Geometry: final body of the model. Coordinates: model frame, mm. A direction names the side the tool comes from. Round coordinates to 2 decimals unless told otherwise and drop trailing zeros. Loops run counter-clockwise (first coordinate to the right, second up) from the corner with the lowest first, then second, coordinate; pieces in that order, holes last. Notation, with made-up numbers: (-37.5, -6.75) - (13.5, -6.75) arc R18 ccw to (13.5, 15.25) - close; hole circle Ø11 at (77.25, -33.75). An arc over 180 degrees is marked (long way). Answer as CSV lines item,"result".
from build123d import *

# Parameters (mm, degrees)
SKETCH_1_R      = 2.1
EXTRUDE_1_DEPTH = 3
SKETCH_2_R      = 14
EXTRUDE_2_DEPTH = 8
SKETCH_3_R      = 11
EXTRUDE_3_DEPTH = 3
FILLET_1_R      = 2
FILLET_2_R      = 1


with BuildPart() as part:
    # 草图1 → 凸台-拉伸1 (new body)
    with BuildSketch(Plane.XY):
        with BuildLine():
            Line((-22.192307692, 4.213250442), (-8.346153846, 13.061076371))
            ThreePointArc((-8.346153846, 13.061076371), (0, 15.5), (8.346153846, 13.061076371))
            Line((8.346153846, 13.061076371), (22.192307692, 4.213250442))
            ThreePointArc((22.192307692, 4.213250442), (24.5, 0), (22.192307692, -4.213250442))
            Line((22.192307692, -4.213250442), (8.346153846, -13.061076371))
            ThreePointArc((8.346153846, -13.061076371), (0, -15.5), (-8.346153846, -13.061076371))
            Line((-8.346153846, -13.061076371), (-22.192307692, -4.213250442))
            ThreePointArc((-22.192307692, -4.213250442), (-24.5, 0), (-22.192307692, 4.213250442))
        make_face()
        with Locations((-19.5, 0)):
            Circle(SKETCH_1_R, mode=Mode.SUBTRACT)
        with Locations((19.5, 0)):
            Circle(SKETCH_1_R, mode=Mode.SUBTRACT)
    extrude(amount=EXTRUDE_1_DEPTH)

    # 草图2 → 凸台-拉伸2 (add)
    with BuildSketch(Plane.XY.offset(3)):
        Circle(SKETCH_2_R)
    extrude(amount=EXTRUDE_2_DEPTH)

    # 草图3 → 凸台-拉伸3 (add)
    with BuildSketch(Plane.XY.offset(11)):
        Circle(SKETCH_3_R)
    extrude(amount=EXTRUDE_3_DEPTH)

    # 草图4 → 切除-旋转1 (revolve, cut)
    with BuildSketch(Plane(origin=(0, 0, 0), x_dir=(0, 0, -1), z_dir=(1, 0, 0))):
        with BuildLine():
            Line((-18, 0), (-4, 0))
            ThreePointArc((-4, 0), (-11, 7), (-18, 0))
        make_face()
    revolve(axis=Axis((0, 0, 18), (0, 0, -1)), mode=Mode.SUBTRACT)

    # 圆角1
    fillet_1_edges = [part.edges().sort_by_distance(p)[0] for p in [
        (-14, 0, 11),
    ]]
    fillet(fillet_1_edges, radius=FILLET_1_R)

    # 圆角2
    fillet_2_edges = [part.edges().sort_by_distance(p)[0] for p in [
        (-11, 0, 14),
    ]]
    fillet(fillet_2_edges, radius=FILLET_2_R)


solid = part.part
(1) Access query for faces 1 (the face through (12.932, -5.362, 5.958)), 2 (the face through (0, 0, 0)). Directions: +Z, -Z, +X, -X, +Y, -Y. A direction counts if a zero-diameter tool reaches every point of the face in a straight line with its end or side. Return the directions, or none.
Findings below:
face 1,"+Z"
face 2,"-Z, +X, -X, +Y, -Y"
(2) Section A-A (z = 2.5). Output: boundary loops of the cut face in (x, y), and give its area (3 significant figures).
Findings below:
outline,"(-22.19, -4.21) - (-8.35, -13.06) arc R15.5 ccw to (8.35, -13.06) - (22.19, -4.21) arc R5 ccw to (22.19, 4.21) - (8.35, 13.06) arc R15.5 ccw to (-8.35, 13.06) - (-22.19, 4.21) arc R5 ccw to start; hole circle Ø4.2 at (-19.5, 0); hole circle Ø4.2 at (19.5, 0)"
area,"969 mm2"
(3) Section B-B (x = -19.5). Output: boundary loops of the cut face in (y, z).
Findings below:
outline,"(-5.93, 0) - (-2.1, 0) - (-2.1, 3) - (-5.93, 3) - close; (2.1, 0) - (5.93, 0) - (5.93, 3) - (2.1, 3) - close"
(4) Pin query (flat end, axial travel): P1, Ø1, axis at x = -11, z = 6.5, coming from the -Y side; P2, Ø5.5, axis at x = 19.5, y = 0, coming from the +Z side; P3, Ø3, axis at y = -10, z = 10, coming from the -X side; P4, Ø4, axis at x = -19.5, y = 0, coming from the -Z side. Return the tip coordinate at first contact, or that it passes through.
Findings below:
P1,"y = -9.26"
P2,"z = 3"
P3,"x = -10.98"
P4,"through"
(5) Material intervals for line 1 along Y through (x, z) = (-19.5, 1.7); line 2 along Z through (x, y) = (-15, 7); line 3 along X through (y, z) = (-4.5, 11.25), sorted ascending.
Findings below:
line 1,"-5.93 to -2.1, 2.1 to 5.93"
line 2,"0 to 3"
line 3,"-10.04 to -5.36, 5.36 to 10.04"
(6) Draft query along Y for faces 3 (the face through (-2.38, -10.74, 11.99)), 4 (the face through (21.503, 0.631, 1.479)), 5 (the face through (-17.497, 0.631, 1.479)), 6 (the face through (0.1, -15.5, 1.5)). Return one class per face: pulls with the +Y half, pulls with the -Y half, needs draft (parallel to the pull), parting line crosses it, or undercut.
Findings below:
face 3,"parting line crosses it"
face 4,"undercut"
face 5,"undercut"
face 6,"pulls with the -Y half"
(7) Section D-D (z = 5.75). Output: boundary loops of the cut face in (x, y), and give its area (3 significant figures).
Findings below:
outline,"circle Ø28 at (0, 0); hole circle Ø9.26 at (0, 0)"
area,"548 mm2"
(8) Section C-C (y = 0). Output: boundary loops of the cut face in (x, z).
Findings below:
outline,"(-24.5, 0) - (-21.6, 0) - (-21.6, 3) - (-24.5, 3) - close; (-17.4, 0) - (17.4, 0) - (17.4, 3) - (14, 3) - (14, 9) arc R2 ccw to (12, 11) - (11, 11) - (11, 13) arc R1 ccw to (10, 14) - (6.32, 14) arc R7 cw (long way) to (-6.32, 14) - (-10, 14) arc R1 ccw to (-11, 13) - (-11, 11) - (-12, 11) arc R2 ccw to (-14, 9) - (-14, 3) - (-17.4, 3) - close; (21.6, 0) - (24.5, 0) - (24.5, 3) - (21.6, 3) - close"
